```python
from build123d import *

# Parameters (mm, degrees)
SCHIZZO1_W                             = 20
SCHIZZO1_H                             = 19.7
ESTRUSIONE_ESTRUSIONE1_DEPTH           = 3
FORO_SVASATO_PER_VITE_M2_2_D           = 2.4
FORO_SVASATO_PER_VITE_M2_2_CSINK_D     = 4.4
FORO_SVASATO_PER_VITE_M2_2_CSINK_ANGLE = 90


with BuildPart() as part:
    # Schizzo1 → Estrusione-Estrusione1 (new body)
    with BuildSketch(Plane.XY):
        with Locations((10, 9.85)):
            Rectangle(SCHIZZO1_W, SCHIZZO1_H)
    extrude(amount=ESTRUSIONE_ESTRUSIONE1_DEPTH)

    # Foro svasato per Vite M2-2 (through all)
    with Locations(Plane.XY.offset(3)):
        with Locations((5, 9.85), (15, 9.85)):
            CounterSinkHole(FORO_SVASATO_PER_VITE_M2_2_D / 2, FORO_SVASATO_PER_VITE_M2_2_CSINK_D / 2, counter_sink_angle=FORO_SVASATO_PER_VITE_M2_2_CSINK_ANGLE)


solid = part.part
```
The listing builds one solid part. Answer for the finished solid, in the listing's coordinates (mm). Coordinates: 2 decimals unless noted, no trailing zeros. Loops run counter-clockwise (first coordinate to the right, second up) from the corner with the lowest first, then second, coordinate; pieces in that order, holes last. Notation, with made-up numbers: (64, -28.5) - (103, -28.5) arc R24 cw to (103, 7.5) - close; hole circle Ø1 at (-37.75, 79). An arc over 180 degrees is marked (long way). Write item = value, one per line.
1) Find the intervals of material crossed by line 1 along X through (y, z) = (9.85, 0.9); line 2 along Y through (x, z) = (15, 1.65); line 3 along Z through (x, y) = (14.5, 8), in increasing order.
Responses:
line_1 = 0 to 3.8, 6.2 to 13.8, 16.2 to 20
line_2 = 0 to 8.65, 11.05 to 19.7
line_3 = 0 to 2.72
2) Section C-C (z = 1) is taken. Determine the outline of the cut face in (x, y).
Responses:
outline = (0, 0) - (20, 0) - (20, 19.7) - (0, 19.7) - close; hole circle Ø2.4 at (5, 9.85); hole circle Ø2.4 at (15, 9.85)
3) Section B-B (y = 9.85) is taken. Determine the outline of the cut face in (x, z), plus the area to 3 significant figures.
Responses:
outline = (0, 0) - (3.8, 0) - (3.8, 2) - (2.8, 3) - (0, 3) - close; (6.2, 0) - (13.8, 0) - (13.8, 2) - (12.8, 3) - (7.2, 3) - (6.2, 2) - close; (16.2, 0) - (20, 0) - (20, 3) - (17.2, 3) - (16.2, 2) - close
area = 43.6 mm^2
4) Section A-A (x = 15) is taken. Determine the outline of the cut face in (y, z).
Responses:
outline = (0, 0) - (8.65, 0) - (8.65, 2) - (7.65, 3) - (0, 3) - close; (11.05, 0) - (19.7, 0) - (19.7, 3) - (12.05, 3) - (11.05, 2) - close
5) Section D-D (z = 2.3) is taken. Determine the outline of the cut face in (x, y).
Responses:
outline = (0, 0) - (20, 0) - (20, 19.7) - (0, 19.7) - close; hole circle Ø3 at (5, 9.85); hole circle Ø3 at (15, 9.85)
6) Determine the mould class of faces 1 (the face through (10, 0, 1)), 2 (the face through (13.855, 10.21, 0.986)), 3 (the face through (10, 10, 0)) for opening direction Y: pulls with the +Y half, pulls with the -Y half, needs draft (parallel to the pull), parting line crosses it, or undercut.
Responses:
face_1 = pulls with the -Y half
face_2 = undercut
face_3 = needs draft
